Read the model definition and answer for the solid it produces. Units are mm, in the model's axes. Face numbers are marked on the shaded views. A direction names the side the tool comes from. Round coordinates to 2 decimals unless told otherwise and drop trailing zeros. Order: outer loops, then holes, each group sorted by start corner. A loop starts at its lowest first (then second) coordinate and runs counter-clockwise, first axis right, second up. Notation, with made-up numbers: M 10,67 L 38,67 A31 ccw 38,98 Z; hole C 62.5,-20.75 d8. An arc over 180 degrees is marked long. Answer as CSV lines item,"result".
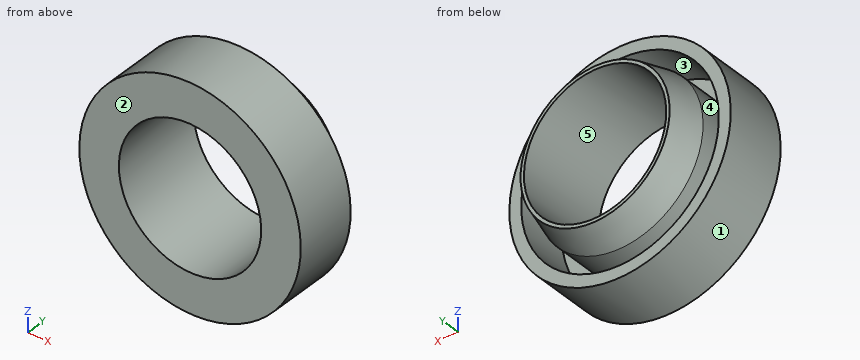
```python
from build123d import *

# Parameters (mm, degrees)
SKETCH1_R           = 14
BOSS_EXTRUDE1_DEPTH = 12
CUT_EXTRUDE1_REACH  = 25.152
SKETCH2_R           = 9
SKETCH3_R           = 12.5
SKETCH3_R_2         = 10.5
CUT_EXTRUDE2_DEPTH  = 10.5
SKETCH4_R           = 14
SKETCH4_R_2         = 12.5
CUT_EXTRUDE3_DEPTH  = 4
CHAMFER1_SIZE       = 4
CHAMFER1_SIZE2      = 1.07179677


with BuildPart() as part:
    # Sketch1 → Boss-Extrude1 (new body)
    with BuildSketch(Plane(origin=(0, 0, 0), x_dir=(1, 0, 0), z_dir=(0, 1, 0))):
        with Locations(Location((0, 0, 0), (0, 0, 270))):
            Circle(SKETCH1_R)
    extrude(amount=BOSS_EXTRUDE1_DEPTH)

    # Sketch2 → Cut-Extrude1 (cut, up to next)
    with BuildSketch(Plane(origin=(0, 12, 0), x_dir=(1, 0, 0), z_dir=(0, 1, 0)), mode=Mode.PRIVATE) as cut_extrude1_sk1:
        with Locations(Location((0, 0, 0), (0, 0, 270))):
            Circle(SKETCH2_R)
    cut_extrude1_tool1 = extrude(cut_extrude1_sk1.sketch, amount=-CUT_EXTRUDE1_REACH, mode=Mode.PRIVATE) & part.part
    add(cut_extrude1_tool1.solids().sort_by_distance((0, 12, 0))[0], mode=Mode.SUBTRACT)

    # Sketch3 → Cut-Extrude2 (cut)
    with BuildSketch(Plane(origin=(0, 12, 0), x_dir=(1, 0, 0), z_dir=(0, 1, 0))):
        with Locations(Location((0, 0, 0), (0, 0, 270))):
            Circle(SKETCH3_R)
        with Locations(Location((0, 0, 0), (0, 0, 270))):
            Circle(SKETCH3_R_2, mode=Mode.SUBTRACT)
    extrude(amount=-CUT_EXTRUDE2_DEPTH, mode=Mode.SUBTRACT)

    # Sketch4 → Cut-Extrude3 (cut)
    with BuildSketch(Plane(origin=(0, 12, 0), x_dir=(1, 0, 0), z_dir=(0, 1, 0))):
        with Locations(Location((0, 0, 0), (0, 0, 270))):
            Circle(SKETCH4_R)
        with Locations(Location((0, 0, 0), (0, 0, 270))):
            Circle(SKETCH4_R_2, mode=Mode.SUBTRACT)
    extrude(amount=-CUT_EXTRUDE3_DEPTH, mode=Mode.SUBTRACT)

    # Chamfer1
    chamfer1_edges = [part.edges().sort_by_distance(p)[0] for p in [
        (0, 12, -10.5),
    ]]
    chamfer1_side = [part.faces().sort_by_distance(p)[0] for p in [
        (0, 6.75, -10.5),
    ]]
    chamfer(chamfer1_edges, length=CHAMFER1_SIZE, length2=CHAMFER1_SIZE2, reference=chamfer1_side[0])


solid = part.part
```
Item 1: Flat-ended cylindrical pins translate along their axes: pin 1 (6 mm diameter, centred on x = 5.5, y = 5.5, fed in from +Z) (3 decimals); pin 2 (1.5 mm diameter, centred on x = -6.5, z = 9.5, fed in from +Y); pin 3 (1.5 mm diameter, centred on x = -1.5, y = 6.5, fed in from -Z). Find the tip coordinate at first contact, or state that the pin passes through.
Ans:
pin 1,"z = 13.775"
pin 2,"y = 1.5"
pin 3,"z = -13.98"
Item 2: Find the intervals of material crossed by probe 1 along X at (y, z) = (5.5, 0); probe 2 along X at (y, z) = (2, 7.5); probe 3 along Z at (x, y) = (6.75, 6.25), in increasing order. Write a range as [from, to].
Ans:
probe 1,"[-14, -12.5], [-10.5, -9], [9, 10.5], [12.5, 14]"
probe 2,"[-11.82, -10], [-7.35, -4.97], [4.97, 7.35], [10, 11.82]"
probe 3,"[-12.27, -10.52], [-8.04, -5.95], [5.95, 8.04], [10.52, 12.27]"
Item 3: A cutting plane is placed at D-D, the plane z = 11.75. Determine the outline of the cut face in (x, y).
Ans:
outline,"M -7.61,0 L 7.61,0 L 7.61,8 L 4.26,8 L 4.26,1.5 L -4.26,1.5 L -4.26,8 L -7.61,8 Z"
Item 4: Determine the mould class of the marked faces 1, 2 and 3 for opening direction Z: +Z half, -Z half, draft (parallel to the pull), parting line (faces both ways), or undercut.
Ans:
face 1,"parting line"
face 2,"draft"
face 3,"undercut"
Item 5: A cutting plane is placed at C-C, the plane y = 3. Determine the outline of the cut face in (x, z).
Ans:
outline,"C 0,0 d28; C 0,0 d21; hole C 0,0 d25; hole C 0,0 d18"
Item 6: A tool of negligible diameter and unlimited length cuts with its end or side. For the marked faces 4 and 5, from which of +Z, -Z, +X, -X, +Y, -Y can it reach the whole face along a straight path? Write none if from no direction.
Ans:
face 4,"+Y"
face 5,"+Y, -Y"
Item 7: A cutting plane is placed at B-B, the plane z = 0. Determine the outline of the cut face in (x, y).
Ans:
outline,"M -14,0 L -9,0 L -9,12 L -9.43,12 L -10.5,8 L -10.5,1.5 L -12.5,1.5 L -12.5,8 L -14,8 Z; M 9,0 L 14,0 L 14,8 L 12.5,8 L 12.5,1.5 L 10.5,1.5 L 10.5,8 L 9.43,12 L 9,12 Z"
Item 8: A cutting plane is placed at A-A, the plane x = 0. Determine the outline of the cut face in (y, z), and give its area (3 significant figures).
Ans:
outline,"M 0,-14 L 8,-14 L 8,-12.5 L 1.5,-12.5 L 1.5,-10.5 L 8,-10.5 L 12,-9.43 L 12,-9 L 0,-9 Z; M 0,9 L 12,9 L 12,9.43 L 8,10.5 L 1.5,10.5 L 1.5,12.5 L 8,12.5 L 8,14 L 0,14 Z"
area,"61.7 mm2"
